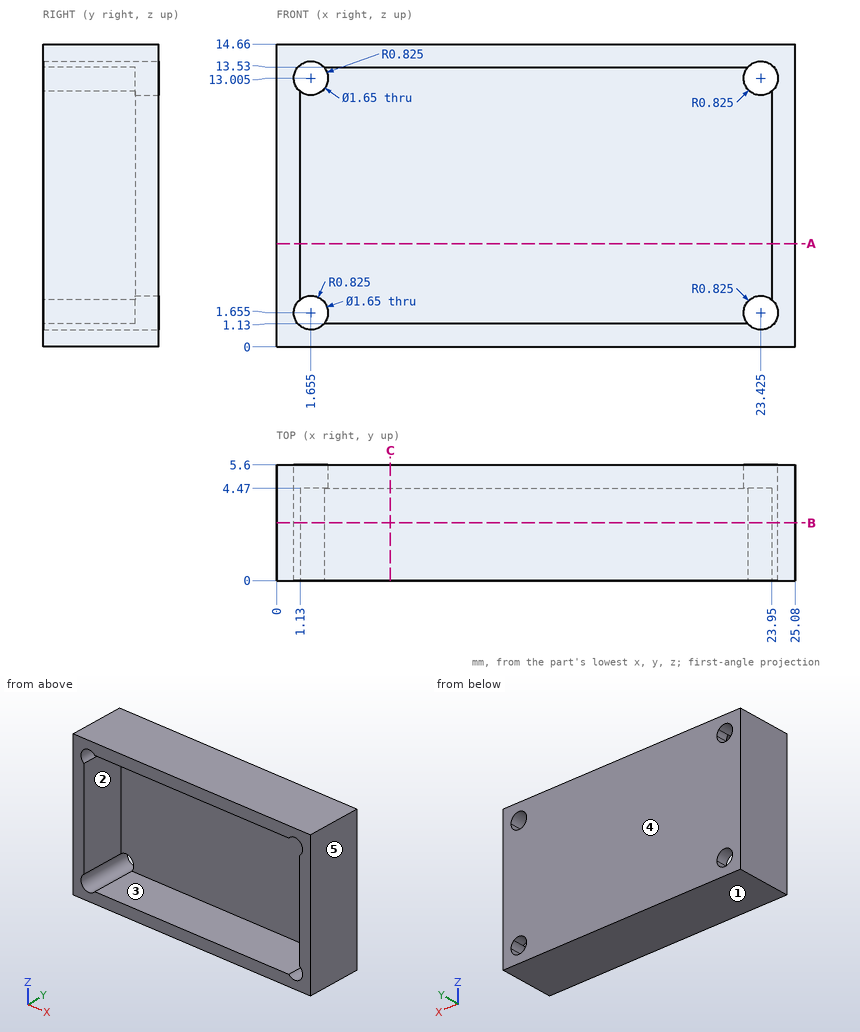
Study the drawing (mm; zero at the part's minimum x, y, z) and answer. A direction names the side the tool comes from. Coordinates: 2 decimals unless noted, no trailing zeros. Write each loop counter-clockwise with the first axis right and the second up, starting at its lowest first coordinate (ties: lowest second). Pieces come first, ordered by that corner, then holes. Notation, with made-up numbers: (-6.5, 75.5) - (14.5, 75.5) arc R18 ccw to (14.5, 85.5) - close; hole circle Ø10 at (58.5, 68). An arc over 180 degrees is marked (long way). One line per item, written item: value.
1) Find section C-C (x = 5.5). Give the vertices of the cut face in (y, z).
Geometry check:
outline: (0, 0) - (5.6, 0) - (5.6, 14.66) - (0, 14.66) - (0, 13.53) - (4.47, 13.53) - (4.47, 1.13) - (0, 1.13) - close
2) Each of these flat-tipped pins is pushed along its axis until it touches: pin 1 Ø1 at (x, y) = (3.5, 3.5) entering from -Z; pin 2 Ø4 at (x, z) = (13.5, 10.5) entering from -Y. Where does it stop, or does it pass through?
Geometry check:
pin 1: stops at z = 0
pin 2: stops at y = 4.47
3) Consider line 1 along Z through (x, y) = (9.5, 2.7); line 2 along X through (y, z) = (0.4, 2.75); line 3 along X through (y, z) = (4.8, 2). Determine where each line is inside the solid, lowest interval first. Write a range as from..to.
Geometry check:
line 1: z = 0..1.13, 13.53..14.66
line 2: x = 0..1.13, 23.95..25.08
line 3: x = 0..0.91, 2.4..22.68, 24.17..25.08
4) Find section A-A (z = 5). Give the vertices of the cut face in (x, y).
Geometry check:
outline: (0, 0) - (1.13, 0) - (1.13, 4.47) - (23.95, 4.47) - (23.95, 0) - (25.08, 0) - (25.08, 5.6) - (0, 5.6) - close
5) A tool of negligible diameter and unlimited length cuts with its end or side. For the marked faces 1 and 2, from which of +Z, -Z, +X, -X, +Y, -Y can it reach the whole face along a straight path? Write none if from no direction.
Geometry check:
face 1: -Z, +X, -X, +Y, -Y
face 2: -Y
6) Find section B-B (y = 2.8). Give the vertices of the cut face in (x, z) (3 decimals), and give its area (3 significant figures).
Geometry check:
outline: (0, 0) - (25.08, 0) - (25.08, 14.66) - (0, 14.66) - close; hole (1.13, 2.291) arc R0.825 ccw (long way) to (2.291, 1.13) - (22.789, 1.13) arc R0.825 ccw (long way) to (23.95, 2.291) - (23.95, 12.369) arc R0.825 ccw (long way) to (22.789, 13.53) - (2.291, 13.53) arc R0.825 ccw (long way) to (1.13, 12.369) - close
area: 82.6 mm2
7) For a pull along X with two mould halves and no side action, classify the marked faces 3, 4 and 5 as pulls with the +X half, pulls with the -X half, needs draft (parallel to the pull), parting line crosses it, or undercut.
Geometry check:
face 3: undercut
face 4: needs draft
face 5: pulls with the +X half
